For this review, take the finished solid that the model builds, in its own axes (mm). A direction names the side the tool comes from. Coordinates: 2 decimals unless noted, no trailing zeros. Loops run counter-clockwise (first coordinate to the right, second up) from the corner with the lowest first, then second, coordinate; pieces in that order, holes last. Notation, with made-up numbers: (57, 13) -> (113, 13) arc R20 ccw to (113, 52) -> close; hole circle Ø9 at (57.5, 29.25). An arc over 180 degrees is marked (long way). Answer in a Markdown table with one row per item.
from build123d import *

# Parameters (mm, degrees)
LINKFRAME_R         = 40
BOSS_EXTRUDE1_DEPTH = 100
EXTENDEDPRESS_W     = 200
EXTENDEDPRESS_H     = 50
BOSS_EXTRUDE2_DEPTH = 200


with BuildPart() as part:
    # LinkFrame → Boss-Extrude1 (new body)
    with BuildSketch(Plane(origin=(0, 0, 0), x_dir=(0, 0, -1), z_dir=(1, 0, 0))):
        with BuildLine():
            Line((316.746524862, -249.209808828), (316.746524862, -366.043560924))
            Line((316.746524862, -366.043560924), (366.746524862, -366.043560924))
            Line((366.746524862, -366.043560924), (366.746524862, -416.043560924))
            Line((366.746524862, -416.043560924), (166.746524862, -416.043560924))
            Line((166.746524862, -416.043560924), (166.746524862, -366.043560924))
            Line((166.746524862, -366.043560924), (216.746524862, -366.043560924))
            Line((216.746524862, -366.043560924), (216.746524862, -249.209808828))
            ThreePointArc((216.746524862, -249.209808828), (266.746524862, -156.043560924), (316.746524862, -249.209808828))
        make_face()
        with Locations((266.746524862, -216.043560924)):
            Circle(LINKFRAME_R, mode=Mode.SUBTRACT)
    extrude(amount=BOSS_EXTRUDE1_DEPTH)

    # ExtendedPress → Boss-Extrude2 (add, symmetric)
    with BuildSketch(Plane(origin=(0, 0, 0), x_dir=(0, 0, -1), z_dir=(1, 0, 0))):
        with Locations((266.746524862, -391.043560924)):
            Rectangle(EXTENDEDPRESS_W, EXTENDEDPRESS_H)
    extrude(amount=BOSS_EXTRUDE2_DEPTH, both=True)


solid = part.part
Item 1: For L1, parallel to Y at x = -141.5, z = -184; L2, parallel to X at y = -177, z = -288; L3, parallel to Z at x = 20.5, y = -218.5, list the stretches that pass through material, from the lowest coordinate up.
Worked answers:
| item | result |
|---|---|
| L1 | -416.04 to -366.04 |
| L2 | 0 to 100 |
| L3 | -326.7 to -306.67, -226.82 to -206.8 |
Item 2: The part is to be moulded in two halves that separate along Z. For faces 1 (the cylindrical face through (49.3, -156.07, -264.94)), 2 (the cylindrical face through (49.3, -214.285, -226.785)), 3 (the flat face through (3, -391, -366.747)), say which applies: +Z half, -Z half, draft (parallel to the pull), parting line (faces both ways), or undercut.
Worked answers:
| item | result |
|---|---|
| face 1 | parting line |
| face 2 | undercut |
| face 3 | -Z half |
Item 3: Take a section at D-D, the plane y = -228. State the section outline as (x, z) points, and give its area (3 significant figures).
Worked answers:
| item | result |
|---|---|
| outline | (0, -325.54) -> (100, -325.54) -> (100, -304.92) -> (0, -304.92) -> close; (0, -228.58) -> (100, -228.58) -> (100, -207.95) -> (0, -207.95) -> close |
| area | 4,130 mm² |
Item 4: Take a section at C-C, the plane x = 20. State the section outline as (y, z) points.
Worked answers:
| item | result |
|---|---|
| outline | (-416.04, -366.75) -> (-366.04, -366.75) -> (-366.04, -316.75) -> (-249.21, -316.75) arc R60 ccw (long way) to (-249.21, -216.75) -> (-366.04, -216.75) -> (-366.04, -166.75) -> (-416.04, -166.75) -> close; hole circle Ø80 at (-216.04, -266.75) |
Item 5: Insertion check: pin 1 (3 mm diameter, centred on y = -238, z = -228, fed in from -X); pin 2 (3 mm diameter, centred on x = 98.5, y = -294.5, fed in from +Z); pin 3 (1 mm diameter, centred on x = 34, y = -237.5, fed in from -Z). Each pin has a flat end and moves straight along its axis. Give the tip position at first contact, or say it passes through.
Worked answers:
| item | result |
|---|---|
| pin 1 | x = 0 |
| pin 2 | z = -216.75 |
| pin 3 | z = -322.97 |
Item 6: For faces 4 (the flat face through (49, -307, -316.747)), 5 (the flat face through (200, -391, -265)), 6 (the flat face through (100, -283, -268)), 7 (the flat face through (49, -308, -216.747)), 8 (the flat face through (0, -283, -268)), list the 3-axis set-ups (+Z, -Z, +X, -X, +Y, -Y) from which the entire face can be reached by the end or side of a thin tool; tool diameter is ignored.
Worked answers:
| item | result |
|---|---|
| face 4 | -Z, +X, -X |
| face 5 | +Z, -Z, +X, +Y, -Y |
| face 6 | +Z, -Z, +X, +Y |
| face 7 | +Z, +X, -X |
| face 8 | +Z, -Z, -X, +Y |
Item 7: Take a section at A-A, the plane y = -190.5. State the section outline as (x, z) points, and give its area (3 significant figures).
Worked answers:
| item | result |
|---|---|
| outline | (0, -321.04) -> (100, -321.04) -> (100, -297.53) -> (0, -297.53) -> close; (0, -235.96) -> (100, -235.96) -> (100, -212.46) -> (0, -212.46) -> close |
| area | 4,700 mm² |
Item 8: Take a section at B-B, the plane z = -250.5. State the section outline as (x, y) points (3 decimals), and give its area (3 significant figures).
Worked answers:
| item | result |
|---|---|
| outline | (-200, -416.044) -> (200, -416.044) -> (200, -366.044) -> (100, -366.044) -> (100, -252.596) -> (0, -252.596) -> (0, -366.044) -> (-200, -366.044) -> close; (0, -179.492) -> (100, -179.492) -> (100, -158.285) -> (0, -158.285) -> close |
| area | 33,500 mm² |
